from build123d import *

# Parameters (mm, degrees)
CROQUIS1_R              = 22.5
CROQUIS1_R_2            = 3.96875
CROQUIS1_R_3            = 1.5875
CROQUIS1_W              = 10
CROQUIS1_H              = 3.175
SALIENTE_EXTRUIR1_DEPTH = 3.175


with BuildPart() as part:
    # Croquis1 → Saliente-Extruir1 (new body)
    with BuildSketch(Plane(origin=(0, 0, 0), x_dir=(1, 0, 0), z_dir=(0, 1, 0))):
        Circle(CROQUIS1_R)
        Circle(CROQUIS1_R_2, mode=Mode.SUBTRACT)
        with Locations((0, 7.9375)):
            Circle(CROQUIS1_R_3, mode=Mode.SUBTRACT)
        with Locations((0, -7.9375)):
            Circle(CROQUIS1_R_3, mode=Mode.SUBTRACT)
        with Locations((0, 14.2875)):
            Circle(CROQUIS1_R_3, mode=Mode.SUBTRACT)
        with Locations((0, -14.2875)):
            Circle(CROQUIS1_R_3, mode=Mode.SUBTRACT)
        with Locations((-10, 6.4125)):
            Rectangle(CROQUIS1_W, CROQUIS1_H, mode=Mode.SUBTRACT)
        with Locations((10, 6.4125)):
            Rectangle(CROQUIS1_W, CROQUIS1_H, mode=Mode.SUBTRACT)
        with Locations((-10, -6.4125)):
            Rectangle(CROQUIS1_W, CROQUIS1_H, mode=Mode.SUBTRACT)
        with Locations((10, -6.4125)):
            Rectangle(CROQUIS1_W, CROQUIS1_H, mode=Mode.SUBTRACT)
    extrude(amount=SALIENTE_EXTRUIR1_DEPTH)


solid = part.part
Geometry check sheet. Reference: the model listing, model coordinates, mm. A direction names the side the tool comes from. Give positions to 0.01 mm unless a question says otherwise; leave off trailing zeros. Loops run counter-clockwise (first coordinate to the right, second up) from the corner with the lowest first, then second, coordinate; pieces in that order, holes last.
(1) Section check C-C on x = -11.5. Record the cut outline in (y, z) (3 decimals).
From the geometry:
outline: (0, -19.339) - (3.175, -19.339) - (3.175, -8) - (0, -8) - close; (0, -4.825) - (3.175, -4.825) - (3.175, 4.825) - (0, 4.825) - close; (0, 8) - (3.175, 8) - (3.175, 19.339) - (0, 19.339) - close
(2) Section check D-D on y = 2.25. Count the separate pieces of the cut face and the enclosed holes in it, then the cut area to 3 significant figures.
From the geometry:
separate pieces: 1
enclosed holes: 9
area: 1,380 mm2
(3) Depth check by flat-ended pin: pin 1 Ø1 at (y, z) = (1, -6) entering from -X; pin 2 Ø3 at (x, z) = (0, -7.94) entering from +Y; pin 3 Ø1.6 at (y, z) = (1, -6) entering from -X; pin 4 Ø1 at (x, y) = (12, 1.5) entering from -Z. Enter the tip coordinate at first touch or a pass-through.
From the geometry:
pin 1: stops at x = -21.82
pin 2: passes through
pin 3: stops at x = -21.89
pin 4: stops at z = -19.34
(4) Section check A-A on x = 0. Record the cut outline in (y, z) (3 decimals), then the cut area to 3 significant figures.
From the geometry:
outline: (0, -22.5) - (3.175, -22.5) - (3.175, -15.875) - (0, -15.875) - close; (0, -12.7) - (3.175, -12.7) - (3.175, -9.525) - (0, -9.525) - close; (0, -6.35) - (3.175, -6.35) - (3.175, -3.969) - (0, -3.969) - close; (0, 3.969) - (3.175, 3.969) - (3.175, 6.35) - (0, 6.35) - close; (0, 9.525) - (3.175, 9.525) - (3.175, 12.7) - (0, 12.7) - close; (0, 15.875) - (3.175, 15.875) - (3.175, 22.5) - (0, 22.5) - close
area: 77.4 mm2
(5) Thickness scan on L1, parallel to Z at x = 0, y = 1.8 (3 decimals); L2, parallel to Z at x = -6, y = 1.65 (3 decimals); L3, parallel to X at y = 1.55, z = -7. Record the ranges inside material, lowest first.
From the geometry:
L1: z = -22.5 to -15.875, -12.7 to -9.525, -6.35 to -3.969, 3.969 to 6.35, 9.525 to 12.7, 15.875 to 22.5
L2: z = -21.685 to -8, -4.825 to 4.825, 8 to 21.685
L3: x = -21.38 to -15, -5 to -1.28, 1.28 to 5, 15 to 21.38
(6) Release check for a two-part mould opening along Z. For faces 3 (the flat face through (0, 3.175, 5)), 4 (the cylindrical face through (-0.86, 1.565, 3.874)) record: released by +Z, released by -Z, zero draft, split by the parting line, or undercut.
From the geometry:
face 3: zero draft
face 4: undercut
(7) Section check B-B on z = 0. Record the cut outline in (x, y) (3 decimals).
From the geometry:
outline: (-22.5, 0) - (-3.969, 0) - (-3.969, 3.175) - (-22.5, 3.175) - close; (3.969, 0) - (22.5, 0) - (22.5, 3.175) - (3.969, 3.175) - close
(8) Set-up check for faces 1 (the flat face through (15, 2, -6)), 2 (the flat face through (0, 0, 5)): record each of +Z, -Z, +X, -X, +Y, -Y from which the full face is reachable in a straight line by a thin tool's end or side.
From the geometry:
face 1: +Y, -Y
face 2: +Z, -Z, +X, -X, -Y
